Check sheet for the modelled part. Datum: model origin and axes. Units: mm. A direction names the side the tool comes from. Round coordinates to 2 decimals unless told otherwise and drop trailing zeros. Loops run counter-clockwise (first coordinate to the right, second up) from the corner with the lowest first, then second, coordinate; pieces in that order, holes last. Notation, with made-up numbers: (21, 34.25) - (46, 34.25) arc R31 cw to (46, 59.25) - close; hole circle Ø3 at (4, -20.5). An arc over 180 degrees is marked (long way). Answer in a Markdown table with one row per item. Add a question column.
(1) Access from +Z, -Z, +X, -X, +Y, -Y to the whole of each face (thin tool, end or side, straight path). Record for faces 5 (the cylindrical face through (121.189, -10.965, 276.437)), 6 (the cylindrical face through (-121.189, 10.965, -276.437)), 7 (the cylindrical face through (105.545, -3.543, 289.084)), 8 (the flat face through (-2, 0, 273.25)).
(2) Gauge pin test, flat ends, axial feed: pin 1 (5.5 mm diameter, centred on x = 64.5, y = -1, fed in from +Z); pin 2 (5 mm diameter, centred on x = 133, z = 246.68, fed in from +Y); pin 3 (9 mm diameter, centred on x = -63.5, y = -1.5, fed in from +Z). Record the tip position at first contact, or that the pin passes through.
(3) Cross-section at B-B on z = -27.5. Enter the section's corners in (x, y), then the cut area to 3 significant figures.
(4) Cross-section at A-A on x = 11. Enter the section's corners in (y, z), then the cut area to 3 significant figures.
(5) Thickness scan on line 1 along Z through (x, y) = (60.5, -10.5); line 2 along Z through (x, y) = (-107, -7.5); line 3 along Y through (x, z) = (65, 276.5). Record the ranges inside material, lowest first.
(6) Mould release check, pull along Z, two halves, no side actions. Record for faces 1 (the flat face through (2, 0, -273.25)), 2 (the cylindrical face through (130.979, 0.169, -286.445)), 3 (the cylindrical face through (-130.979, 0.169, 286.445)), 4 (the cylindrical face through (59.955, 0.222, 278.193)): +Z half, -Z half, draft (parallel to the pull), parting line (faces both ways), or undercut.
from build123d import *

# Parameters (mm, degrees)
SKETCH1_W                      = 304.8
SKETCH1_H                      = 609.6
F_1_X2_HDPE_STOCK_DEPTH        = 12.05
BASE_ENCLOSURE_DIMS_DEPTH      = 342.627882352
BASE_ENCLOSURE_DIMS_DEPTH_BACK = 342.627882352
SKETCH2_W                      = 304.8
SKETCH2_H                      = 609.6
SKETCH2_W_2                    = 280
SKETCH2_H_2                    = 590
FILLET1_R                      = 30
SKETCH3_R                      = 3.15
CUT_EXTRUDE4_DEPTH             = 328.422983311
CRVPATTERN1_START              = -13
CRVPATTERN1_OUTLINE_R          = 3.15
CRVPATTERN1_DEPTH              = 26
ORING_GROOVE_DEPTH             = 2.2
CUT_EXTRUDE6_DEPTH             = 328.422983311
CUT_EXTRUDE6_DEPTH_BACK        = 328.422983311
CUT_EXTRUDE7_REACH             = 608.502
SKETCH7_R                      = 5.05
SKETCH7_R_2                    = 7.05
SKETCH8_R                      = 11.25
CUT_EXTRUDE8_DEPTH             = 10
SKETCH9_R                      = 9.25
CUT_EXTRUDE9_DEPTH             = 12


with BuildPart() as part:
    # Sketch1 → 1"x2" HDPE Stock (new, symmetric)
    with BuildSketch(Plane(origin=(0, 0, 0), x_dir=(1, 0, 0), z_dir=(0, 1, 0))):
        Rectangle(SKETCH1_W, SKETCH1_H)
    extrude(amount=F_1_X2_HDPE_STOCK_DEPTH, both=True)

    # Sketch2 → Base Enclosure Dims (cut, two sides: drawn at the far end of the back side and taken through both)
    with BuildSketch(Plane(origin=(0, 12.05, 0), x_dir=(1, 0, 0), z_dir=(0, 1, 0)).offset(-BASE_ENCLOSURE_DIMS_DEPTH_BACK)):
        Rectangle(SKETCH2_W, SKETCH2_H)
        Rectangle(SKETCH2_W_2, SKETCH2_H_2, mode=Mode.SUBTRACT)
    extrude(amount=BASE_ENCLOSURE_DIMS_DEPTH + BASE_ENCLOSURE_DIMS_DEPTH_BACK, mode=Mode.SUBTRACT)

    # Fillet1
    fillet1_edges = [part.edges().sort_by_distance(p)[0] for p in [
        (140, 0, 295),
        (140, 0, -295),
        (-140, 0, -295),
        (-140, 0, 295),
    ]]
    fillet(fillet1_edges, radius=FILLET1_R)

    # Sketch3 → Cut-Extrude4 (cut, symmetric)
    with BuildSketch(Plane(origin=(0, 12.05, 0), x_dir=(1, 0, 0), z_dir=(0, 1, 0))):
        with Locations(Location((0, -288, 0), (0, 0, 270))):
            Circle(SKETCH3_R)
    extrude(amount=CUT_EXTRUDE4_DEPTH, both=True, mode=Mode.SUBTRACT)

    # CrvPattern1: read off the stored shape, not the designer's step
    # CrvPattern1 outline → CrvPattern1 (cut)
    with BuildSketch(Plane(origin=(0, 0, 0), x_dir=(1, 0, 0), z_dir=(0, 1, 0)).offset(CRVPATTERN1_START)):
        with Locations((82.225663103, -288)):
            Circle(CRVPATTERN1_OUTLINE_R)
        with Locations((-82.225663103, -288)):
            Circle(CRVPATTERN1_OUTLINE_R)
        with Locations((-133, -246.67698931)):
            Circle(CRVPATTERN1_OUTLINE_R)
        with Locations((-133, -164.451326207)):
            Circle(CRVPATTERN1_OUTLINE_R)
        with Locations((-133, -82.225663103)):
            Circle(CRVPATTERN1_OUTLINE_R)
        with Locations((-133, 0)):
            Circle(CRVPATTERN1_OUTLINE_R)
        with Locations((-133, 82.225663103)):
            Circle(CRVPATTERN1_OUTLINE_R)
        with Locations((-133, 164.451326207)):
            Circle(CRVPATTERN1_OUTLINE_R)
        with Locations((-133, 246.67698931)):
            Circle(CRVPATTERN1_OUTLINE_R)
        with Locations((-82.225663103, 288)):
            Circle(CRVPATTERN1_OUTLINE_R)
        with Locations((0, 288)):
            Circle(CRVPATTERN1_OUTLINE_R)
        with Locations((82.225663103, 288)):
            Circle(CRVPATTERN1_OUTLINE_R)
        with Locations((133, 246.67698931)):
            Circle(CRVPATTERN1_OUTLINE_R)
        with Locations((133, 164.451326207)):
            Circle(CRVPATTERN1_OUTLINE_R)
        with Locations((133, 82.225663103)):
            Circle(CRVPATTERN1_OUTLINE_R)
        with Locations((133, 0)):
            Circle(CRVPATTERN1_OUTLINE_R)
        with Locations((133, -82.225663103)):
            Circle(CRVPATTERN1_OUTLINE_R)
        with Locations((133, -164.451326207)):
            Circle(CRVPATTERN1_OUTLINE_R)
        with Locations((133, -246.67698931)):
            Circle(CRVPATTERN1_OUTLINE_R)
    extrude(amount=CRVPATTERN1_DEPTH, mode=Mode.SUBTRACT)

    # Sketch5 → Oring Groove (cut)
    with BuildSketch(Plane(origin=(0, 12.05, 0), x_dir=(1, 0, 0), z_dir=(0, 1, 0))):
        with BuildLine():
            Line((-126, 265), (-126, -265))
            ThreePointArc((-126, -265), (-121.313708499, -276.313708499), (-110, -281))
            Line((-110, -281), (110, -281))
            ThreePointArc((110, -281), (121.313708499, -276.313708499), (126, -265))
            Line((126, -265), (126, 265))
            ThreePointArc((126, 265), (121.313708499, 276.313708499), (110, 281))
            Line((110, 281), (-110, 281))
            ThreePointArc((-110, 281), (-121.313708499, 276.313708499), (-126, 265))
        make_face()
        with BuildLine():
            Line((122.25, -265), (122.25, 265))
            ThreePointArc((122.25, 265), (118.66205807, 273.66205807), (110, 277.25))
            Line((110, 277.25), (-110, 277.25))
            ThreePointArc((-110, 277.25), (-118.66205807, 273.66205807), (-122.25, 265))
            Line((-122.25, 265), (-122.25, -265))
            ThreePointArc((-122.25, -265), (-118.66205807, -273.66205807), (-110, -277.25))
            Line((-110, -277.25), (110, -277.25))
            ThreePointArc((110, -277.25), (118.66205807, -273.66205807), (122.25, -265))
        make_face(mode=Mode.SUBTRACT)
    oring_groove = extrude(amount=-ORING_GROOVE_DEPTH, mode=Mode.SUBTRACT)

    # Sketch6 → Cut-Extrude6 (cut, two sides: drawn at the far end of the back side and taken through both)
    with BuildSketch(Plane(origin=(0, 12.05, 0), x_dir=(1, 0, 0), z_dir=(0, 1, 0)).offset(-CUT_EXTRUDE6_DEPTH_BACK)):
        with BuildLine():
            Line((118.25, -265), (118.25, 265))
            ThreePointArc((118.25, 265), (115.833630945, 270.833630945), (110, 273.25))
            Line((110, 273.25), (-110, 273.25))
            ThreePointArc((-110, 273.25), (-115.833630945, 270.833630945), (-118.25, 265))
            Line((-118.25, 265), (-118.25, -265))
            ThreePointArc((-118.25, -265), (-115.833630945, -270.833630945), (-110, -273.25))
            Line((-110, -273.25), (110, -273.25))
            ThreePointArc((110, -273.25), (115.833630945, -270.833630945), (118.25, -265))
        make_face()
    extrude(amount=CUT_EXTRUDE6_DEPTH + CUT_EXTRUDE6_DEPTH_BACK, mode=Mode.SUBTRACT)

    # Mirror1: Oring Groove across plane
    add(oring_groove.mirror(Plane.ZX), mode=Mode.SUBTRACT)

    # Sketch7 → Cut-Extrude7 (cut, up to next)
    with BuildSketch(Plane.XY.offset(295), mode=Mode.PRIVATE) as cut_extrude7_sk1:
        with Locations((-65, 0)):
            Circle(SKETCH7_R)
    cut_extrude7_tool1 = extrude(cut_extrude7_sk1.sketch, amount=-CUT_EXTRUDE7_REACH, mode=Mode.PRIVATE) & part.part
    # Sketch7 → Cut-Extrude7 (cut, up to next)
    with BuildSketch(Plane.XY.offset(295), mode=Mode.PRIVATE) as cut_extrude7_sk2:
        with Locations((-97, 0)):
            Circle(SKETCH7_R_2)
    cut_extrude7_tool2 = extrude(cut_extrude7_sk2.sketch, amount=-CUT_EXTRUDE7_REACH, mode=Mode.PRIVATE) & part.part
    # Sketch7 → Cut-Extrude7 (cut, up to next)
    with BuildSketch(Plane.XY.offset(295), mode=Mode.PRIVATE) as cut_extrude7_sk3:
        with Locations((97, 0)):
            Circle(SKETCH7_R)
    cut_extrude7_tool3 = extrude(cut_extrude7_sk3.sketch, amount=-CUT_EXTRUDE7_REACH, mode=Mode.PRIVATE) & part.part
    # Sketch7 → Cut-Extrude7 (cut, up to next)
    with BuildSketch(Plane.XY.offset(295), mode=Mode.PRIVATE) as cut_extrude7_sk4:
        with Locations((65, 0)):
            Circle(SKETCH7_R)
    cut_extrude7_tool4 = extrude(cut_extrude7_sk4.sketch, amount=-CUT_EXTRUDE7_REACH, mode=Mode.PRIVATE) & part.part
    add(cut_extrude7_tool1.solids().sort_by_distance((-65, 0, 295))[0], mode=Mode.SUBTRACT)
    add(cut_extrude7_tool2.solids().sort_by_distance((-97, 0, 295))[0], mode=Mode.SUBTRACT)
    add(cut_extrude7_tool3.solids().sort_by_distance((97, 0, 295))[0], mode=Mode.SUBTRACT)
    add(cut_extrude7_tool4.solids().sort_by_distance((65, 0, 295))[0], mode=Mode.SUBTRACT)

    # Sketch8 → Cut-Extrude8 (cut)
    with BuildSketch(Plane.XY.offset(295)):
        with Locations((-97, 0)):
            Circle(SKETCH8_R)
    extrude(amount=-CUT_EXTRUDE8_DEPTH, mode=Mode.SUBTRACT)

    # Sketch9 → Cut-Extrude9 (cut)
    with BuildSketch(Plane.XY.offset(295)):
        with Locations((-65, 0)):
            Circle(SKETCH9_R)
        with Locations((65, 0)):
            Circle(SKETCH9_R)
        with Locations((97, 0)):
            Circle(SKETCH9_R)
    extrude(amount=-CUT_EXTRUDE9_DEPTH, mode=Mode.SUBTRACT)


solid = part.part
Answers:
| question | item | result |
|---|---|---|
| 1 | face 5 | -Y |
| 1 | face 6 | +Y |
| 1 | face 7 | +Z |
| 1 | face 8 | +Y, -Y |
| 2 | pin 1 | stops at z = -273.25 |
| 2 | pin 2 | passes through |
| 2 | pin 3 | stops at z = 283 |
| 3 | outline | (-140, -12.05) - (-126, -12.05) - (-126, -9.85) - (-122.25, -9.85) - (-122.25, -12.05) - (-118.25, -12.05) - (-118.25, 12.05) - (-122.25, 12.05) - (-122.25, 9.85) - (-126, 9.85) - (-126, 12.05) - (-140, 12.05) - close; (118.25, -12.05) - (122.25, -12.05) - (122.25, -9.85) - (126, -9.85) - (126, -12.05) - (140, -12.05) - (140, 12.05) - (126, 12.05) - (126, 9.85) - (122.25, 9.85) - (122.25, 12.05) - (118.25, 12.05) - close |
| 3 | area | 1,020 mm^2 |
| 4 | outline | (-12.05, -295) - (12.05, -295) - (12.05, -281) - (9.85, -281) - (9.85, -277.25) - (12.05, -277.25) - (12.05, -273.25) - (-12.05, -273.25) - (-12.05, -277.25) - (-9.85, -277.25) - (-9.85, -281) - (-12.05, -281) - close; (-12.05, 273.25) - (12.05, 273.25) - (12.05, 277.25) - (9.85, 277.25) - (9.85, 281) - (12.05, 281) - (12.05, 295) - (-12.05, 295) - (-12.05, 281) - (-9.85, 281) - (-9.85, 277.25) - (-12.05, 277.25) - close |
| 4 | area | 1,020 mm^2 |
| 5 | line 1 | z = -295 to -281, -277.25 to -273.25, 273.25 to 277.25, 281 to 295 |
| 5 | line 2 | z = -295 to -273.25, 273.25 to 295 |
| 5 | line 3 | y = -12.05 to -5.05, 5.05 to 12.05 |
| 6 | face 1 | undercut |
| 6 | face 2 | -Z half |
| 6 | face 3 | +Z half |
| 6 | face 4 | draft |
